Autodesk Inventor part; units mm, degrees
ref_plane "YZ Plane" through (0, 0, 0) normal (1, 0, 0) x (0, 1, 0)
ref_plane "XZ Plane" through (0, 0, 0) normal (0, 1, 0) x (-1, 0, 0)
ref_plane "XY Plane" through (0, 0, 0) normal (0, 0, 1) x (1, 0, 0)
sketch "Sketch1" plane through (0, 0, 0) normal (0, 0, 1) x (1, 0, 0)
  line L0 (-1152.525, 0) -> (1152.525, 0)
  line L1 (-19.05, 0) -> (19.05, 0)
  line L2 (-19.05, 0) -> (-19.05, 1828.8)
  line L3 (19.05, 0) -> (19.05, 1828.8)
  line L4 (19.05, 1828.8) -> (-19.05, 1828.8)
  line L5 (1152.525, 0) -> (1152.525, 1828.8)
  line L6 (1152.525, 1828.8) -> (19.05, 1828.8)
  line L7 (-1152.525, 0) -> (-1152.525, 1828.8)
  line L8 (-1152.525, 1828.8) -> (-19.05, 1828.8)
  line L9 (-1152.525, 1828.8) -> (-19.05, 0)
  line L10 (19.05, 0) -> (1152.525, 1828.8)
  line L11 (-56.8317, -23.4168) -> (18.7317, 23.4168)
  line L12 (-1190.3067, 1805.3832) -> (-1114.7433, 1852.2168)
  line L13 (-1190.3067, 1805.3832) -> (-56.8317, -23.4168)
  line L14 (18.7317, 23.4168) -> (-1114.7433, 1852.2168)
  line L15 (0, 1828.8) -> (0, 0)
  point P0 (-19.05, 84.3755)
  point P1 (-1100.2298, 1828.8)
  point P2 (-1152.525, 1744.4245)
  point P3 (-71.3452, 0)
  dimension "d0" = 2305.05
  dimension "d1" = 38.1
  dimension "d2" = 1828.8
  dimension "d3" = 1828.8
  dimension "d4" = 1828.8
  dimension "d5" = 1828.8
  dimension "d6" = 88.9
  dimension "d7" = 88.9
extrude "Extrusion1" add sketch "Sketch1" along normal blind 38.1 contours L9 L8 L14 L2 | L0 L13 L7 L9
properties part number "S_2x4x84.708"
Could you check a few things on this model? Use its own coordinates, in mm. Give positions to 0.01 mm unless a question says otherwise; leave off trailing zeros. Order: outer loops, then holes, each group sorted by start corner. A loop starts at its lowest first (then second) coordinate and runs counter-clockwise, first axis right, second up.
1. For pin 1 (10 mm diameter, centred on x = -347.5, z = 4.5, fed in from -Y); pin 2 (12 mm diameter, centred on y = 414, z = 25.5, fed in from -X); pin 3 (3 mm diameter, centred on x = -838, z = 7, fed in from -Y), each with a flat end and sliding along its axis, tell me the tip position at first contact or that it passes through.
Answers below:
pin 1: stops at y = 437.49
pin 2: stops at x = -331.66
pin 3: stops at y = 1234.54
2. Suppose I cut it at B-B (x = -1036.5). Write out the boundary of the cut face in (y, z).
Answers below:
outline: (1557.22, 0) - (1725.98, 0) - (1725.98, 38.1) - (1557.22, 38.1) - close
3. I need wall thicknesses on L1, parallel to Y at x = -70, z = 35; L2, parallel to X at y = 1526, z = 3.5; L3, parallel to Y at x = -958, z = 15. Which ranges of each line are inside material? Lowest first, please.
Answers below:
L1: y = 0 to 166.58
L2: x = -1017.15 to -912.56
L3: y = 1430.57 to 1599.32
4. Suppose I cut it at C-C (y = 546.5). Write out the boundary of the cut face in (x, z), plus the area to 3 significant figures.
Answers below:
outline: (-410.06, 0) - (-305.47, 0) - (-305.47, 38.1) - (-410.06, 38.1) - close
area: 3,980 mm2
